```python
from build123d import *

# Parameters (mm, degrees)
CROQUIS1_R              = 10
SALIENTE_EXTRUIR1_DEPTH = 1.5
CROQUIS2_R              = 10
CROQUIS2_R_2            = 8
SALIENTE_EXTRUIR2_DEPTH = 15
CORTAR_EXTRUIR2_REACH   = 22.616
CROQUIS4_R              = 0.95
CROQUIS5_W              = 3
CROQUIS5_H              = 1.5
CORTAR_EXTRUIR3_DEPTH   = 15
CROQUIS6_R              = 3
CROQUIS6_R_2            = 1.45
SALIENTE_EXTRUIR3_DEPTH = 2


with BuildPart() as part:
    # Croquis1 → Saliente-Extruir1 (new body)
    with BuildSketch(Plane.XY):
        Circle(CROQUIS1_R)
    extrude(amount=SALIENTE_EXTRUIR1_DEPTH)

    # Croquis2 → Saliente-Extruir2 (add)
    with BuildSketch(Plane.XY.offset(1.5)):
        Circle(CROQUIS2_R)
        Circle(CROQUIS2_R_2, mode=Mode.SUBTRACT)
    extrude(amount=SALIENTE_EXTRUIR2_DEPTH)

    # Croquis4 → Cortar-Extruir2 (cut, up to next)
    with BuildSketch(Plane.XY.offset(1.5), mode=Mode.PRIVATE) as cortar_extruir2_sk1:
        with Locations((-5.999300536, -0.09161372)):
            Circle(CROQUIS4_R)
    cortar_extruir2_tool1 = extrude(cortar_extruir2_sk1.sketch, amount=-CORTAR_EXTRUIR2_REACH, mode=Mode.PRIVATE) & part.part
    # Croquis4 → Cortar-Extruir2 (cut, up to next)
    with BuildSketch(Plane.XY.offset(1.5), mode=Mode.PRIVATE) as cortar_extruir2_sk2:
        with Locations((-0.09161372, 5.999300536)):
            Circle(CROQUIS4_R)
    cortar_extruir2_tool2 = extrude(cortar_extruir2_sk2.sketch, amount=-CORTAR_EXTRUIR2_REACH, mode=Mode.PRIVATE) & part.part
    # Croquis4 → Cortar-Extruir2 (cut, up to next)
    with BuildSketch(Plane.XY.offset(1.5), mode=Mode.PRIVATE) as cortar_extruir2_sk3:
        with Locations((5.999300536, 0.09161372)):
            Circle(CROQUIS4_R)
    cortar_extruir2_tool3 = extrude(cortar_extruir2_sk3.sketch, amount=-CORTAR_EXTRUIR2_REACH, mode=Mode.PRIVATE) & part.part
    # Croquis4 → Cortar-Extruir2 (cut, up to next)
    with BuildSketch(Plane.XY.offset(1.5), mode=Mode.PRIVATE) as cortar_extruir2_sk4:
        with Locations((0.09161372, -5.999300536)):
            Circle(CROQUIS4_R)
    cortar_extruir2_tool4 = extrude(cortar_extruir2_sk4.sketch, amount=-CORTAR_EXTRUIR2_REACH, mode=Mode.PRIVATE) & part.part
    add(cortar_extruir2_tool1.solids().sort_by_distance((-5.999301, -0.091614, 1.5))[0], mode=Mode.SUBTRACT)
    add(cortar_extruir2_tool2.solids().sort_by_distance((-0.091614, 5.999301, 1.5))[0], mode=Mode.SUBTRACT)
    add(cortar_extruir2_tool3.solids().sort_by_distance((5.999301, 0.091614, 1.5))[0], mode=Mode.SUBTRACT)
    add(cortar_extruir2_tool4.solids().sort_by_distance((0.091614, -5.999301, 1.5))[0], mode=Mode.SUBTRACT)

    # Croquis5 → Cortar-Extruir3 (cut)
    with BuildSketch(Plane.XY.offset(16.5)):
        with Locations((0, 8)):
            Rectangle(CROQUIS5_W, CROQUIS5_H)
    extrude(amount=-CORTAR_EXTRUIR3_DEPTH, mode=Mode.SUBTRACT)

    # Croquis6 → Saliente-Extruir3 (add)
    with BuildSketch(Plane.XY.offset(1.5)):
        with BuildLine():
            Line((1.5, 7.858116823), (1.5, 8.75))
            Line((1.5, 8.75), (-1.5, 8.75))
            Line((-1.5, 8.75), (-1.5, 7.858116823))
            ThreePointArc((-1.5, 7.858116823), (0, -8), (1.5, 7.858116823))
        make_face()
        Circle(CROQUIS6_R, mode=Mode.SUBTRACT)
        with Locations((-0.09161372, 5.999300536)):
            Circle(CROQUIS6_R_2, mode=Mode.SUBTRACT)
        with Locations((5.999300536, 0.09161372)):
            Circle(CROQUIS6_R_2, mode=Mode.SUBTRACT)
        with Locations((-5.999300536, -0.09161372)):
            Circle(CROQUIS6_R_2, mode=Mode.SUBTRACT)
        with Locations((0.09161372, -5.999300536)):
            Circle(CROQUIS6_R_2, mode=Mode.SUBTRACT)
    extrude(amount=SALIENTE_EXTRUIR3_DEPTH)


solid = part.part
```
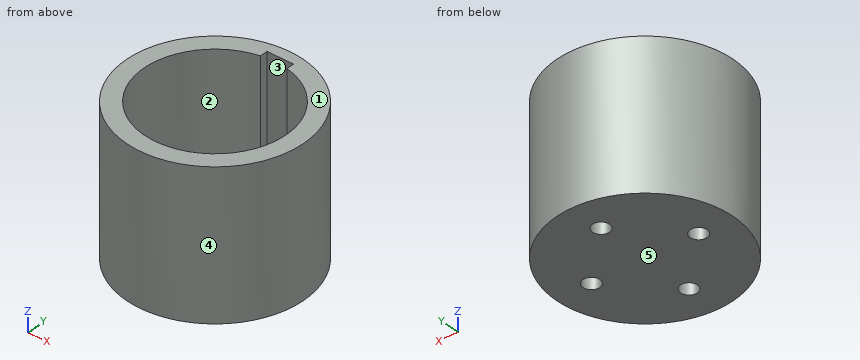
The listing builds one solid part. Answer for the finished solid, in the listing's coordinates (mm). Face numbers are marked on the shaded views. A direction names the side the tool comes from. Give positions to 0.01 mm unless a question says otherwise; leave off trailing zeros. Loops run counter-clockwise (first coordinate to the right, second up) from the corner with the lowest first, then second, coordinate; pieces in that order, holes last. Notation, with made-up numbers: (10.5, -33.5) - (22.5, -33.5) arc R26 cw to (22.5, 0.5) - close; hole circle Ø3 at (-5, 83.5). An arc over 180 degrees is marked (long way). Answer as CSV lines item,"result". Start each with the question number.
Item 1: A cutting plane is placed at B-B on y = -6.5. Determine the outline of the cut face in (x, z).
Item 2: The mould has two halves that part along Y. Classify the marked faces 3, 4 and 5: +Y half, -Y half, draft (parallel to the pull), parting line (faces both ways), or undercut.
Item 3: A cutting plane is placed at A-A on z = 7.5. Determine the outline of the cut face in (x, y).
Item 4: Each of these flat-tipped pins is pushed along its axis until it touches: pin 1 (1.5 mm diameter, centred on y = -1, z = 3.5, fed in from -X); pin 2 (5 mm diameter, centred on x = -4, y = 1.5, fed in from +Z); pin 3 (2.5 mm diameter, centred on x = -6, y = -0.09, fed in from +Z). Where does it stop, or does it pass through?
Item 5: A cutting plane is placed at C-C on x = 0. Determine the outline of the cut face in (y, z).
Item 6: Find the intervals of material crossed by line 1 (Z direction, x = 7.5, y = -1.75); line 2 (X direction, y = 2.75, z = 4); line 3 (Z direction, x = -5, y = 0.5), in increasing order. Write a range as from..to.
Item 7: For the marked faces 1 and 2, determine the directions among +Z, -Z, +X, -X, +Y, -Y from which every point of the face is accessible in a straight line to the end or side of a thin tool.
Item 8: A cutting plane is placed at D-D on y = -0.5. Determine the outline of the cut face in (x, z), then the cut area to 3 significant figures.
Found:
1,outline,"(-7.6, 0) - (-0.72, 0) - (-0.72, 1.5) - (-1.27, 1.5) - (-1.27, 3.5) - (-4.66, 3.5) - (-4.66, 16.5) - (-7.6, 16.5) - close; (0.9, 0) - (7.6, 0) - (7.6, 16.5) - (4.66, 16.5) - (4.66, 3.5) - (1.45, 3.5) - (1.45, 1.5) - (0.9, 1.5) - close"
2,face 3,"undercut"
2,face 4,"parting line"
2,face 5,"draft"
3,outline,"circle Ø20 at (0, 0); hole (-1.5, 7.86) arc R8 ccw (long way) to (1.5, 7.86) - (1.5, 8.75) - (-1.5, 8.75) - close"
4,pin 1,"stops at x = -10"
4,pin 2,"stops at z = 3.5"
4,pin 3,"stops at z = 1.5"
5,outline,"(-10, 0) - (-6.94, 0) - (-6.94, 1.5) - (-7.45, 1.5) - (-7.45, 3.5) - (-8, 3.5) - (-8, 16.5) - (-10, 16.5) - close; (-5.05, 0) - (5.05, 0) - (5.05, 1.5) - (4.55, 1.5) - (4.55, 3.5) - (3, 3.5) - (3, 1.5) - (-3, 1.5) - (-3, 3.5) - (-4.55, 3.5) - (-4.55, 1.5) - (-5.05, 1.5) - close; (6.94, 0) - (10, 0) - (10, 16.5) - (8.75, 16.5) - (8.75, 3.5) - (7.45, 3.5) - (7.45, 1.5) - (6.94, 1.5) - close"
6,line 1,"z = 0..3.5"
6,line 2,"x = -9.61..-7.51, 7.51..9.61"
6,line 3,"z = 0..1.5"
7,face 1,"+Z, +X, -X, +Y, -Y"
7,face 2,"+Z"
8,outline,"(-9.99, 0) - (-6.86, 0) - (-6.86, 1.5) - (-7.39, 1.5) - (-7.39, 3.5) - (-7.98, 3.5) - (-7.98, 16.5) - (-9.99, 16.5) - close; (-5.14, 0) - (5.26, 0) - (5.26, 1.5) - (4.68, 1.5) - (4.68, 3.5) - (2.96, 3.5) - (2.96, 1.5) - (-2.96, 1.5) - (-2.96, 3.5) - (-4.61, 3.5) - (-4.61, 1.5) - (-5.14, 1.5) - close; (6.74, 0) - (9.99, 0) - (9.99, 16.5) - (7.98, 16.5) - (7.98, 3.5) - (7.32, 3.5) - (7.32, 1.5) - (6.74, 1.5) - close"
8,area,"94.5 mm^2"
